For this review, take the finished solid that the model builds, in its own axes (mm). A direction names the side the tool comes from. Round coordinates to 2 decimals unless told otherwise and drop trailing zeros. Loops run counter-clockwise (first coordinate to the right, second up) from the corner with the lowest first, then second, coordinate; pieces in that order, holes last.
1) Take a section at C-C (y = -1.75). State the section outline as (x, z) points.
2) Take a section at B-B (x = 4). State the section outline as (y, z) points, then the cut area to 3 significant figures.
3) Wall thickness on L1, parallel to X at y = -1.6, z = -0.95; L2, parallel to X at y = 0.4, z = 0.95; L3, parallel to Z at x = 4, y = -0.1: over which ranges is each line inside the solid? List them lowest first.
4) Mouldability with a two-part tool opening along Y and no side actions: class faces 1 (the flat face through (0, 2, 0)), 2 (the cylindrical face through (-0.986, -0.596, -2.685)), 3 (the flat face through (-1.26, -0.86, 0.51)) as pulls with the +Y half, pulls with the -Y half, needs draft (parallel to the pull), parting line crosses it, or undercut.
5) Insertion check: pin 1 (2 mm diameter, centred on x = 2, y = -2, fed in from -Z); pin 2 (2 mm diameter, centred on x = 6, z = 0.5, fed in from -Y). Each pin has a flat end and moves straight along its axis. Give the tip position at first contact, or say it passes through.
6) Tool access review of faces 4 (the flat face through (-1.26, -0.87, -0.49)), 5 (the cylindrical face through (3.95, -1.5, 0.07)), 6 (the flat face through (-2, 0, -1.2)): name each direction out of +Z, -Z, +X, -X, +Y, -Y from which nothing blocks a thin tool from reaching the whole face with its end or side.
7) Take a section at A-A (z = 2.2). State the section outline as (x, y) points, then the cut area to 3 significant figures.
Autodesk Inventor part; units mm, degrees
ref_plane "bolt_XY" through (0, 0, 0) normal (1, 0, 0) x (0, 0, -1)
ref_plane "bolt_YZ" through (0, 0, 0) normal (0, 0, -1) x (0, 1, 0)
ref_plane "bolt_ZX" through (0, 0, 0) normal (0, 1, 0) x (1, 0, 0)
sketch "Sketch_1" plane through (0, 0, 0) normal (0, 0, 1) x (1, 0, 0)
  line L0 (8, 0) -> (-2, 0)
  line L1 (-2, 0) -> (-2, 2.75)
  line L2 (-2, 2.75) -> (0, 2.75)
  line L3 (0, 2.75) -> (0, 1.6)
  arc A0 (0, 1.6) -> (0.1, 1.5) centre (0.1, 1.6) ccw
  line L4 (0.1, 1.5) -> (7.6935, 1.5)
  line L5 (7.6935, 1.5) -> (8, 1.1935)
  line L6 (8, 1.1935) -> (8, 0)
  line L7 (8, 0) -> (-2, 0)
revolve "Revolution1" add sketch "Sketch_1" angle 360 about axis through (8, 0, 0) along (1, 0, 0)
thread "Thread1"
sketch "Sketch2" plane through (-2, 0, 0) normal (-1, 0, 0) x (0, 0, 1)
  point P0 (0, 0)
hole "Hole1" at (-2, 0, 0) direction (1, 0, 0) diameter 2 depth 1.5 tip angle 140
sketch "Sketch_3" plane through (-2, 0, 0) normal (1, 0, 0) x (0, 0, -1)
  line L0 (-1, 0.5774) -> (-1, -0.5774)
  line L1 (-1, -0.5774) -> (0, -1.1547)
  line L2 (0, -1.1547) -> (1, -0.5774)
  line L3 (1, -0.5774) -> (1, 0.5774)
  line L4 (1, 0.5774) -> (0, 1.1547)
  line L5 (0, 1.1547) -> (-1, 0.5774)
extrude "Extrusion1" cut sketch "Sketch_3" along normal blind 1.5
ref_plane "bolt_XY" through (0, 0, 0) normal (1, 0, 0) x (0, 0, -1)
ref_plane "bolt_YZ" through (0, 0, 0) normal (0, 0, -1) x (0, 1, 0)
ref_plane "bolt_ZX" through (0, 0, 0) normal (0, 1, 0) x (1, 0, 0)
ref_plane "bolt_to_nut_XY" through (8, 0, 0) normal (1, 0, 0) x (0, 0, -1)
ref_plane "bolt_to_nut_YZ" through (8, 0, 0) normal (0, 0, -1) x (0, 1, 0)
ref_plane "bolt_to_nut_ZX" through (8, 0, 0) normal (0, 1, 0) x (1, 0, 0)
properties part number "CBS3-8"
Response:
1. outline: (-2, -2.12) - (0, -2.12) - (0, 2.12) - (-2, 2.12) - close
2. outline: circle Ø3 at (0, 0)
2. area: 7.07 mm2
3. L1: x = -2 to 0
3. L2: x = -0.5 to 8
3. L3: z = -1.5 to 1.5
4. face 1: needs draft
4. face 2: parting line crosses it
4. face 3: undercut
5. pin 1: stops at z = -1.12
5. pin 2: stops at y = -1.5
6. face 4: -X
6. face 5: +X
6. face 6: +Z, -Z, -X, +Y, -Y
7. outline: (-2, -1.65) - (0, -1.65) - (0, 1.65) - (-2, 1.65) - close
7. area: 6.60 mm2
